```python
from build123d import *

# Parameters (mm, degrees)
SKETCH1_W           = 50
SKETCH1_H           = 34.7
BOSS_EXTRUDE1_DEPTH = 10
CUT_EXTRUDE1_REACH  = 34.032
SKETCH2_R           = 1.75
SKETCH3_R           = 3
CUT_EXTRUDE2_DEPTH  = 5
SKETCH6_W           = 50
SKETCH6_H           = 10
BOSS_EXTRUDE3_DEPTH = 44.7
BOSS_EXTRUDE4_DEPTH = 8
BOSS_EXTRUDE5_DEPTH = 8
CHAMFER1_SIZE       = 8
CUT_EXTRUDE3_REACH  = 105.292
SKETCH10_R          = 1.75
CHAMFER2_SIZE       = 8


with BuildPart() as part:
    # Sketch1 → Boss-Extrude1 (new body)
    with BuildSketch(Plane(origin=(0, 0, 0), x_dir=(1, 0, 0), z_dir=(0, 1, 0))):
        Rectangle(SKETCH1_W, SKETCH1_H)
    extrude(amount=BOSS_EXTRUDE1_DEPTH)

    # Sketch2 → Cut-Extrude1 (cut, up to next)
    with BuildSketch(Plane(origin=(0, 10, 0), x_dir=(1, 0, 0), z_dir=(0, 1, 0)), mode=Mode.PRIVATE) as cut_extrude1_sk1:
        with Locations(Location((-10, 7.5, 0), (0, 0, 270))):
            Circle(SKETCH2_R)
    cut_extrude1_tool1 = extrude(cut_extrude1_sk1.sketch, amount=-CUT_EXTRUDE1_REACH, mode=Mode.PRIVATE) & part.part
    # Sketch2 → Cut-Extrude1 (cut, up to next)
    with BuildSketch(Plane(origin=(0, 10, 0), x_dir=(1, 0, 0), z_dir=(0, 1, 0)), mode=Mode.PRIVATE) as cut_extrude1_sk2:
        with Locations(Location((10, 7.5, 0), (0, 0, 270))):
            Circle(SKETCH2_R)
    cut_extrude1_tool2 = extrude(cut_extrude1_sk2.sketch, amount=-CUT_EXTRUDE1_REACH, mode=Mode.PRIVATE) & part.part
    # Sketch2 → Cut-Extrude1 (cut, up to next)
    with BuildSketch(Plane(origin=(0, 10, 0), x_dir=(1, 0, 0), z_dir=(0, 1, 0)), mode=Mode.PRIVATE) as cut_extrude1_sk3:
        with Locations(Location((10, -7.5, 0), (0, 0, 270))):
            Circle(SKETCH2_R)
    cut_extrude1_tool3 = extrude(cut_extrude1_sk3.sketch, amount=-CUT_EXTRUDE1_REACH, mode=Mode.PRIVATE) & part.part
    # Sketch2 → Cut-Extrude1 (cut, up to next)
    with BuildSketch(Plane(origin=(0, 10, 0), x_dir=(1, 0, 0), z_dir=(0, 1, 0)), mode=Mode.PRIVATE) as cut_extrude1_sk4:
        with Locations(Location((-10, -7.5, 0), (0, 0, 270))):
            Circle(SKETCH2_R)
    cut_extrude1_tool4 = extrude(cut_extrude1_sk4.sketch, amount=-CUT_EXTRUDE1_REACH, mode=Mode.PRIVATE) & part.part
    add(cut_extrude1_tool1.solids().sort_by_distance((-10, 10, -7.5))[0], mode=Mode.SUBTRACT)
    add(cut_extrude1_tool2.solids().sort_by_distance((10, 10, -7.5))[0], mode=Mode.SUBTRACT)
    add(cut_extrude1_tool3.solids().sort_by_distance((10, 10, 7.5))[0], mode=Mode.SUBTRACT)
    add(cut_extrude1_tool4.solids().sort_by_distance((-10, 10, 7.5))[0], mode=Mode.SUBTRACT)

    # Sketch3 → Cut-Extrude2 (cut)
    with BuildSketch(Plane(origin=(0, 10, 0), x_dir=(1, 0, 0), z_dir=(0, 1, 0))):
        with Locations(Location((-10, 7.5, 0), (0, 0, 270))):
            Circle(SKETCH3_R)
        with Locations(Location((10, 7.5, 0), (0, 0, 270))):
            Circle(SKETCH3_R)
        with Locations(Location((10, -7.5, 0), (0, 0, 270))):
            Circle(SKETCH3_R)
        with Locations(Location((-10, -7.5, 0), (0, 0, 270))):
            Circle(SKETCH3_R)
    extrude(amount=-CUT_EXTRUDE2_DEPTH, mode=Mode.SUBTRACT)

    # Sketch6 → Boss-Extrude3 (add)
    with BuildSketch(Plane.XZ):
        with Locations((0, 22.35)):
            Rectangle(SKETCH6_W, SKETCH6_H)
    extrude(amount=-BOSS_EXTRUDE3_DEPTH)

    # Sketch8 → Boss-Extrude4 (add)
    with BuildSketch(Plane(origin=(25, 0, 0), x_dir=(0, 0, -1), z_dir=(1, 0, 0))):
        Polygon((-27.35, 0), (17.35, 0), (25.85, -8.5), (72.35, -8.5), (72.35, -28.5), (1.15, -28.5), align=None)
    extrude(amount=-BOSS_EXTRUDE4_DEPTH)

    # Sketch9 → Boss-Extrude5 (add)
    with BuildSketch(Plane(origin=(25, 0, 0), x_dir=(0, 0, -1), z_dir=(1, 0, 0))):
        Polygon((-17.35, 44.7), (17.35, 10), (-17.35, 10), align=None)
    boss_extrude5 = extrude(amount=-BOSS_EXTRUDE5_DEPTH)

    # Chamfer1
    chamfer1_edges = [part.edges().sort_by_distance(p)[0] for p in [
        (21, -8.5, -72.35),
    ]]
    chamfer(chamfer1_edges, length=CHAMFER1_SIZE)

    # Mirror1: Boss-Extrude5 across plane
    add(boss_extrude5.mirror(Plane(origin=(0, 0, 0), x_dir=(0, 0, 1), z_dir=(1, 0, 0))))

    # Sketch10 → Cut-Extrude3 (cut, up to next)
    with BuildSketch(Plane(origin=(0, 0, 17.35), x_dir=(-1, 0, 0), z_dir=(0, 0, -1)), mode=Mode.PRIVATE) as cut_extrude3_sk1:
        with Locations((-10, 34.85)):
            Circle(SKETCH10_R)
    cut_extrude3_tool1 = extrude(cut_extrude3_sk1.sketch, amount=-CUT_EXTRUDE3_REACH, mode=Mode.PRIVATE) & part.part
    # Sketch10 → Cut-Extrude3 (cut, up to next)
    with BuildSketch(Plane(origin=(0, 0, 17.35), x_dir=(-1, 0, 0), z_dir=(0, 0, -1)), mode=Mode.PRIVATE) as cut_extrude3_sk2:
        with Locations((10, 34.85)):
            Circle(SKETCH10_R)
    cut_extrude3_tool2 = extrude(cut_extrude3_sk2.sketch, amount=-CUT_EXTRUDE3_REACH, mode=Mode.PRIVATE) & part.part
    # Sketch10 → Cut-Extrude3 (cut, up to next)
    with BuildSketch(Plane(origin=(0, 0, 17.35), x_dir=(-1, 0, 0), z_dir=(0, 0, -1)), mode=Mode.PRIVATE) as cut_extrude3_sk3:
        with Locations((10, 19.85)):
            Circle(SKETCH10_R)
    cut_extrude3_tool3 = extrude(cut_extrude3_sk3.sketch, amount=-CUT_EXTRUDE3_REACH, mode=Mode.PRIVATE) & part.part
    # Sketch10 → Cut-Extrude3 (cut, up to next)
    with BuildSketch(Plane(origin=(0, 0, 17.35), x_dir=(-1, 0, 0), z_dir=(0, 0, -1)), mode=Mode.PRIVATE) as cut_extrude3_sk4:
        with Locations((-10, 19.85)):
            Circle(SKETCH10_R)
    cut_extrude3_tool4 = extrude(cut_extrude3_sk4.sketch, amount=-CUT_EXTRUDE3_REACH, mode=Mode.PRIVATE) & part.part
    add(cut_extrude3_tool1.solids().sort_by_distance((10, 34.85, 17.35))[0], mode=Mode.SUBTRACT)
    add(cut_extrude3_tool2.solids().sort_by_distance((-10, 34.85, 17.35))[0], mode=Mode.SUBTRACT)
    add(cut_extrude3_tool3.solids().sort_by_distance((-10, 19.85, 17.35))[0], mode=Mode.SUBTRACT)
    add(cut_extrude3_tool4.solids().sort_by_distance((10, 19.85, 17.35))[0], mode=Mode.SUBTRACT)

    # Chamfer2
    chamfer2_edges = [part.edges().sort_by_distance(p)[0] for p in [
        (25, 44.7, 22.35),
        (-25, 44.7, 22.35),
        (-25, 0, 5),
    ]]
    chamfer(chamfer2_edges, length=CHAMFER2_SIZE)


solid = part.part
```
Part model, mm, in its own coordinate system. A direction names the side the tool comes from. Coordinates: 2 decimals unless noted, no trailing zeros. Order: outer loops, then holes, each group sorted by start corner. A loop starts at its lowest first (then second) coordinate and runs counter-clockwise, first axis right, second up. Notation, with made-up numbers: (-27.75, -16) -> (15.25, -16) arc R22 cw to (15.25, 9) -> close; hole circle Ø9 at (-22, 14.25). An arc over 180 degrees is marked (long way). Put each result on its own line as item: value. Start each with the question number.
(1) Band-saw the part on B-B (z = 7.5). Give the cut face in (x, y), then the cut area to 3 significant figures.
(2) Which spindle directions (+Z, -Z, +X, -X, +Y, -Y) get a long thin tool onto all of the face, cutting with end or side? Do faces 1 (the face through (10, 5, -5.5)), 2 (the face through (21, -8.5, -45)), 3 (the face through (0, 22, 27.35)), 4 (the face through (11.5, 2.5, -6.6)), 5 (the face through (17, 20, 7)). Say none if no direction does.
(3) Band-saw the part on A-A (x = -10). Count the separate pieces of the cut face and the enclosed holes in it, then the cut area to 3 significant figures.
(4) Pin check, flat tips, straight feed: pin 1 Ø4.5 at (x, y) = (-10, 19.85) entering from -Z; pin 2 Ø3 at (x, z) = (10, -7.5) entering from -Y; pin 3 Ø6 at (x, z) = (-19.5, -10) entering from -Y; pin 4 Ø6.5 at (x, z) = (-11, 9) entering from +Y. Stop position of each tip, or through.
(5) Band-saw the part on D-D (y = 19.85). Give the cut face in (x, z), then the cut area to 3 significant figures.
(6) Probe line 1 along X through (y, z) = (8, -7.5); line 2 along Y through (x, z) = (10, 19.75); line 3 along X through (y, z) = (1.5, -7.5). List the from-to ranges inside material, lowest first. Write a range as [from, to].
(7) Mould opens along Z. For faces 6 (the face through (0, 5, -17.35)), 7 (the face through (11.5, 2.5, 8.4)), 8 (the face through (17, -17, -23)) say: pulls with the +Z half, pulls with the -Z half, needs draft (parallel to the pull), parting line crosses it, or undercut.
(8) Band-saw the part on C-C (y = 34.85). Give the cut face in (x, z).
Determined:
1. outline: (-25, 8) -> (-17, 0) -> (-11.75, 0) -> (-11.75, 5) -> (-13, 5) -> (-13, 10) -> (-17, 10) -> (-17, 34.85) -> (-25, 34.85) -> close; (-8.25, 0) -> (8.25, 0) -> (8.25, 5) -> (7, 5) -> (7, 10) -> (-7, 10) -> (-7, 5) -> (-8.25, 5) -> close; (11.75, 0) -> (17, 0) -> (17, -19.85) -> (25, -19.85) -> (25, 34.85) -> (17, 34.85) -> (17, 10) -> (13, 10) -> (13, 5) -> (11.75, 5) -> close
1. area: 929 mm²
2. face 1: +Y
2. face 2: -Z, +X, -X, +Y
2. face 3: +Z, +X, -X, +Y, -Y
2. face 4: +Y, -Y
2. face 5: -Z, +Y
3. separate pieces: 5
3. enclosed holes: 0
3. area: 629 mm²
4. pin 1: stops at z = 17.35
4. pin 2: passes through
4. pin 3: stops at y = 0
4. pin 4: stops at y = 10
5. outline: (-25, -7.5) -> (-17, -7.5) -> (-17, 17.35) -> (-11.75, 17.35) -> (-11.75, 27.35) -> (-25, 27.35) -> close; (-8.25, 17.35) -> (8.25, 17.35) -> (8.25, 27.35) -> (-8.25, 27.35) -> close; (11.75, 17.35) -> (17, 17.35) -> (17, -7.5) -> (25, -7.5) -> (25, 27.35) -> (11.75, 27.35) -> close
5. area: 828 mm²
6. line 1: x = [-25, -13], [-7, 7], [13, 25]
6. line 2: y = [0, 18.1], [21.6, 33.1], [36.6, 44.7]
6. line 3: x = [-18.5, -11.75], [-8.25, 8.25], [11.75, 25]
7. face 6: pulls with the -Z half
7. face 7: undercut
7. face 8: needs draft
8. outline: (-25, 7.5) -> (-17, 7.5) -> (-17, 17.35) -> (-11.75, 17.35) -> (-11.75, 27.35) -> (-25, 27.35) -> close; (-8.25, 17.35) -> (8.25, 17.35) -> (8.25, 27.35) -> (-8.25, 27.35) -> close; (11.75, 17.35) -> (17, 17.35) -> (17, 7.5) -> (25, 7.5) -> (25, 27.35) -> (11.75, 27.35) -> close
